```python
from build123d import *

# Parameters (mm, degrees)
SKETCH1_R           = 2.25
BOSS_EXTRUDE1_DEPTH = 45
SKETCH2_R           = 2.25
SKETCH2_R_2         = 2
CUT_EXTRUDE1_DEPTH  = 4
SKETCH3_R           = 2.25
SKETCH3_R_2         = 2
CUT_EXTRUDE2_DEPTH  = 5


with BuildPart() as part:
    # Sketch1 → Boss-Extrude1 (new body, symmetric)
    with BuildSketch(Plane(origin=(0, 0, 0), x_dir=(0, 0, -1), z_dir=(1, 0, 0))):
        Circle(SKETCH1_R)
    extrude(amount=BOSS_EXTRUDE1_DEPTH, both=True)

    # Sketch2 → Cut-Extrude1 (cut)
    with BuildSketch(Plane(origin=(45, 0, 0), x_dir=(0, 0, -1), z_dir=(1, 0, 0))):
        Circle(SKETCH2_R)
        Circle(SKETCH2_R_2, mode=Mode.SUBTRACT)
    extrude(amount=-CUT_EXTRUDE1_DEPTH, mode=Mode.SUBTRACT)

    # Sketch3 → Cut-Extrude2 (cut)
    with BuildSketch(Plane.ZY.offset(45)):
        Circle(SKETCH3_R)
        Circle(SKETCH3_R_2, mode=Mode.SUBTRACT)
    extrude(amount=-CUT_EXTRUDE2_DEPTH, mode=Mode.SUBTRACT)


solid = part.part
```
Model file for the job. Use its own axes, mm. A direction names the side the tool comes from. Give positions to 0.01 mm unless a question says otherwise; leave off trailing zeros. Loops run counter-clockwise (first coordinate to the right, second up) from the corner with the lowest first, then second, coordinate; pieces in that order, holes last. Notation, with made-up numbers: M 77.5,-3 L 126.5,-3 A12 ccw 126.5,1 Z; hole C 1,79 d8. An arc over 180 degrees is marked long. Use one line per item in the form item = value.
Item 1: Drill centre lines: L1, parallel to Z at x = -28, y = 0.2; L2, parallel to Z at x = -11.5, y = -1.05; L3, parallel to X at y = 1.75, z = 1.35. Where is each one in solid material? Low to high.
Filled in:
L1 = -2.24 to 2.24
L2 = -1.99 to 1.99
L3 = -40 to 41
Item 2: Slice it at A-A on z = 0.2. List the corners of the cut face in (x, y).
Filled in:
outline = M -45,-1.99 L -40,-1.99 L -40,-2.24 L 41,-2.24 L 41,-1.99 L 45,-1.99 L 45,1.99 L 41,1.99 L 41,2.24 L -40,2.24 L -40,1.99 L -45,1.99 Z
Item 3: Which spindle directions (+Z, -Z, +X, -X, +Y, -Y) get a long thin tool onto all of the face, cutting with end or side? Do faces 1 (the cylindrical face through (43, -2, 0)), 2 (the cylindrical face through (-43, -2, 0)), 3 (the cylindrical face through (1.07, 2.23, 0.29)). Say none if no direction does.
Filled in:
face_1 = +X
face_2 = -X
face_3 = +X, -X
Item 4: Slice it at B-B on x = -14.5. List the corners of the cut face in (y, z).
Filled in:
outline = C 0,0 d4.5
